Design review of the part built by this model. Coordinates are the model's own, in mm. A direction names the side the tool comes from. Coordinates: 2 decimals unless noted, no trailing zeros. Loops run counter-clockwise (first coordinate to the right, second up) from the corner with the lowest first, then second, coordinate; pieces in that order, holes last.
Q1. Add section B-B on x = -3.5. Give the boundary of the cut face in (y, z).
Q2. Machinability: for faces 4 (the face through (3.4, -12.6, 5)), 5 (the face through (-3.556, -0.878, 21.954)), 6 (the face through (3, -15.7, 3.5)), which of the approach directions +Z, -Z, +X, -X, +Y, -Y give a long, thin tool a straight path to every point of the face, cutting with its end or side? Answer none if there is none.
Q3. Wall thickness on probe 1 along X at (y, z) = (-14, 0.85); probe 2 along Y at (x, z) = (-1, 18); probe 3 along Y at (x, z) = (1.75, 7): over which ranges is each line inside the solid? List them lowest first.
Q4. Add section C-C on y = -14.5. Give the boundary of the cut face in (x, z), and give its area (3 significant figures).
Q5. For P1, Ø4, axis at x = 0, y = -14, coming from the -Z side; P2, Ø5.5, axis at x = 1, y = -13.5, coming from the +Z side; P3, Ø4, axis at x = -1, z = 13.5, coming from the +Y side; P4, Ø3.5, axis at x = -1.5, y = 13.5, coming from the +Z side, all flat-tipped, find the tip position at first contact; note any pin that passes through.
Q6. Add section D-D on z = 19.5. Give the boundary of the cut face in (x, y), and give its area (3 significant figures).
Q7. Add section A-A on y = 0. Give the boundary of the cut face in (x, z), and give its area (3 significant figures).
Q8. Draft analysis for pull direction Y (two halves, no side actions). For faces 1 (the face through (0, -20, 3)), 2 (the face through (3.4, 15.4, 5)), 3 (the face through (0, -10.55, 3)), state which applies: released by +Y, released by -Y, zero draft, split by the parting line, or undercut.
```python
from build123d import *

# Parameters (mm, degrees)
PAD_DEPTH            = 7.5
POCKET_DEPTH         = 3.1
SKETCH002_R          = 2.5
POCKET001_DEPTH      = 126.020998
SKETCH003_R          = 4.05
POCKET002_DEPTH      = 8
POCKET003_DEPTH      = 20.001
POCKET003_DEPTH_BACK = -20.001


with BuildPart() as part:
    # Sketch → Pad (new body, symmetric)
    with BuildSketch(Plane.YZ):
        with BuildLine():
            Line((-20, 0), (20, 0))
            Line((20, 0), (20, 5))
            Line((20, 5), (8, 5))
            Line((8, 5), (8, 18))
            ThreePointArc((8, 18), (0, 26), (-8, 18))
            Line((-8, 18), (-8, 5))
            Line((-8, 5), (-20, 5))
            Line((-20, 5), (-20, 0))
        make_face()
    extrude(amount=PAD_DEPTH, both=True)

    # Sketch001 (on Face7 of Pad) → Pocket (cut)
    with BuildSketch(Plane(origin=(0, 0, 5), x_dir=(0, -1, 0), z_dir=(0, 0, 1))):
        Polygon((-10.55, 1.991858), (-14, 3.983717), (-17.45, 1.991858), (-17.45, -1.991858), (-14, -3.983717), (-10.55, -1.991858), align=None)
    pocket = extrude(amount=-POCKET_DEPTH, mode=Mode.SUBTRACT)

    # Sketch002 (on Face1 of Pocket) → Pocket001 (cut, through all)
    with BuildSketch(Plane.YX):
        with Locations((14, 0)):
            Circle(SKETCH002_R)
    pocket001 = extrude(amount=-POCKET001_DEPTH, mode=Mode.SUBTRACT)

    # Mirrored: Pocket, Pocket001 across XZ
    add(pocket.mirror(Plane.XZ), mode=Mode.SUBTRACT)
    add(pocket001.mirror(Plane.XZ), mode=Mode.SUBTRACT)

    # Sketch003 (on Face3 of Mirrored) → Pocket002 (cut)
    with BuildSketch(Plane(origin=(-7.5, 0, 0), x_dir=(0, 1, 0), z_dir=(-1, 0, 0))):
        with Locations((0, -18)):
            Circle(SKETCH003_R)
    extrude(amount=-POCKET002_DEPTH, mode=Mode.SUBTRACT)

    # Sketch004 → Pocket003 (cut, two sides)
    with BuildSketch(Plane.XZ) as pocket003_sk:
        Polygon((7.5, 5), (2.5, 26), (7.5, 26), align=None)
    extrude(amount=-POCKET003_DEPTH, mode=Mode.SUBTRACT)
    extrude(pocket003_sk.sketch, amount=-POCKET003_DEPTH_BACK, mode=Mode.SUBTRACT)


solid = part.part
```
Entries:
1. outline: (-20, 0) - (20, 0) - (20, 5) - (14.84, 5) - (14.84, 1.9) - (13.16, 1.9) - (13.16, 5) - (8, 5) - (8, 18) arc R8 ccw to (-8, 18) - (-8, 5) - (-13.16, 5) - (-13.16, 1.9) - (-14.84, 1.9) - (-14.84, 5) - (-20, 5) - close; hole circle Ø8.1 at (0, 18)
2. face 4: +Z, +X, -X, -Y
2. face 5: -X
2. face 6: +Z
3. probe 1: x = -7.5 to -2.5, 2.5 to 7.5
3. probe 2: y = -8 to -4.05, 4.05 to 8
3. probe 3: y = -8 to 8
4. outline: (-7.5, 0) - (-2.45, 0) - (-2.45, 1.9) - (-3.7, 1.9) - (-3.7, 5) - (-7.5, 5) - close; (2.45, 0) - (7.5, 0) - (7.5, 5) - (3.7, 5) - (3.7, 1.9) - (2.45, 1.9) - close
4. area: 42.8 mm2
5. P1: passes through
5. P2: stops at z = 5
5. P3: stops at y = 8
5. P4: stops at z = 1.9
6. outline: (-7.5, -7.86) - (4.05, -7.86) - (4.05, 7.86) - (-7.5, 7.86) - (-7.5, 3.76) - (0.5, 3.76) - (0.5, -3.76) - (-7.5, -3.76) - close
6. area: 121 mm2
7. outline: (-7.5, 0) - (7.5, 0) - (7.5, 5) - (2.5, 26) - (-7.5, 26) - (-7.5, 22.05) - (0.5, 22.05) - (0.5, 13.95) - (-7.5, 13.95) - close
7. area: 273 mm2
8. face 1: released by -Y
8. face 2: zero draft
8. face 3: undercut
